Here's how the part is built. I have some questions about the finished solid (model axes, mm). Face numbers are marked on the shaded views. A direction names the side the tool comes from. Round coordinates to 2 decimals unless told otherwise and drop trailing zeros. Write each loop counter-clockwise with the first axis right and the second up, starting at its lowest first coordinate (ties: lowest second). Pieces come first, ordered by that corner, then holes. Notation, with made-up numbers: (60, 1) -> (118, 1) arc R9 cw to (118, 8) -> close; hole circle Ø11 at (6, 88.5). An arc over 180 degrees is marked (long way). Answer in a Markdown table with one row per item.
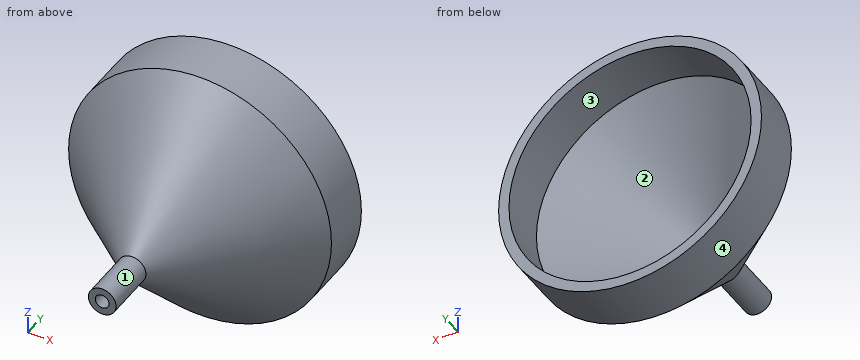
from build123d import *


with BuildPart() as part:
    # basis → roteren (revolve)
    with BuildSketch(Plane.XY, mode=Mode.PRIVATE) as roteren_sk:
        Polygon((-2, 0), (-2, 15), (-36, 49), (-36, 64), (-33, 64), (-33, 50.242640687), (0, 17.242640687), (0, 0), align=None)
    revolve(roteren_sk.sketch.rotate(Axis((2, 0, 0), (0, 1, 0)), 180), axis=Axis((2, 0, 0), (0, 1, 0)))


solid = part.part
1) I want a section at D-D, the plane y = 34. List the corners of the cut face in (x, z) for me, and give its area (3 significant figures).
Response:
| item | result |
|---|---|
| outline | circle Ø46 at (2, 0); hole circle Ø37.51 at (2, 0) |
| area | 557 mm^2 |
2) We'd pull the mould along Z, two halves only. Please class the marked faces 1 and 2: +Z half, -Z half, draft (parallel to the pull), parting line (faces both ways), or undercut.
Response:
| item | result |
|---|---|
| face 1 | parting line |
| face 2 | undercut |
3) Which directions (+Z, -Z, +X, -X, +Y, -Y) give clear straight access to the entire face, cutting with the end or side of a thin tool? Please do the marked faces 3 and 4.
Response:
| item | result |
|---|---|
| face 3 | +Y |
| face 4 | +Y, -Y |
4) I need wall thicknesses on line 1 (Z direction, x = 2, y = 5.5); line 2 (X direction, y = 6.5, z = -1.5); line 3 (Z direction, x = 14, y = 36). Which ranges of each line are inside material? Lowest first, please. Write a range as [from, to].
Response:
| item | result |
|---|---|
| line 1 | z = [-4, -2], [2, 4] |
| line 2 | x = [-1.71, 0.68], [3.32, 5.71] |
| line 3 | z = [-21.93, -16.94], [16.94, 21.93] |
5) I want a section at C-C, the plane y = 21. List the corners of the cut face in (x, z) for me, and give its area (3 significant figures).
Response:
| item | result |
|---|---|
| outline | circle Ø20 at (2, 0); hole circle Ø11.51 at (2, 0) |
| area | 210 mm^2 |
6) I want a section at B-B, the plane x = 2. List the corners of the cut face in (y, z) for me, and give its area (3 significant figures).
Response:
| item | result |
|---|---|
| outline | (0, -4) -> (15, -4) -> (49, -38) -> (64, -38) -> (64, -35) -> (50.24, -35) -> (17.24, -2) -> (0, -2) -> close; (0, 2) -> (17.24, 2) -> (50.24, 35) -> (64, 35) -> (64, 38) -> (49, 38) -> (15, 4) -> (0, 4) -> close |
| area | 435 mm^2 |
7) For pin 1 (3 mm diameter, centred on y = 30, z = 9.5, fed in from +X); pin 2 (3 mm diameter, centred on x = 21.5, z = 13, fed in from +Y); pin 3 (8 mm diameter, centred on x = -8, z = -11, fed in from -Y), each with a flat end and sliding along its axis, tell me the tip position at first contact or that it passes through.
Response:
| item | result |
|---|---|
| pin 1 | stops at x = 20.33 |
| pin 2 | stops at y = 40.18 |
| pin 3 | stops at y = 21.87 |
8) I want a section at A-A, the plane z = 0. List the corners of the cut face in (x, y) for me, and give its area (3 significant figures).
Response:
| item | result |
|---|---|
| outline | (-36, 49) -> (-2, 15) -> (-2, 0) -> (0, 0) -> (0, 17.24) -> (-33, 50.24) -> (-33, 64) -> (-36, 64) -> close; (4, 0) -> (6, 0) -> (6, 15) -> (40, 49) -> (40, 64) -> (37, 64) -> (37, 50.24) -> (4, 17.24) -> close |
| area | 435 mm^2 |
